from build123d import *

# Parameters (mm, degrees)
F1_DEPTH = 25
F3_R     = 2.1
F4_DEPTH = 25
F6_R     = 2.2
F7_DEPTH = 25
F8_R     = 4.99999


# Not quite as in the source:
# - a fillet or chamfer is up to 0.001 mm smaller than in the source, because OpenCascade refuses the exact size


with BuildPart() as f1:
    # F0 (on Right) → F1 (new body)
    with BuildSketch(Plane.YZ):
        Polygon((-127.7586124506, 10), (-127.7586124506, 0), (-18.2758603601, 0), (-18.2758603601, 50), (-28.2758603601, 50), (-28.2758603601, 10), align=None)
    extrude(amount=F1_DEPTH)

    # F3 (on face) → F4 (cut)
    with BuildSketch(Plane.XY.offset(10)):
        with Locations((12.5, -117.7586124506)):
            Circle(F3_R)
        with Locations((12.5, -42.7586124506)):
            Circle(F3_R)
    extrude(amount=-F4_DEPTH, mode=Mode.SUBTRACT)

    # F6 (on face) → F7 (cut)
    with BuildSketch(Plane.YZ.offset(25)):
        with Locations((-23.2758603601, 43)):
            Circle(F6_R)
        with Locations((-23.2758603601, 8)):
            Circle(F6_R)
    extrude(amount=-F7_DEPTH, mode=Mode.SUBTRACT)

    # F8 (radius 5 in the source; OpenCascade refuses exactly that, so slightly less here)
    f8_edges = [f1.edges().sort_by_distance(p)[0] for p in [
        (12.5, -28.27586, 10),
        (12.5, -18.27586, 50),
        (12.5, -28.27586, 50),
        (25, -127.758612, 5),
        (0, -127.758612, 5),
    ]]
    fillet(f8_edges, radius=F8_R)


solid = f1.part
Read the model definition and answer for the solid it produces. Units are mm, in the model's axes. A direction names the side the tool comes from. Coordinates: 2 decimals unless noted, no trailing zeros. Order: outer loops, then holes, each group sorted by start corner. A loop starts at its lowest first (then second) coordinate and runs counter-clockwise, first axis right, second up. Notation, with made-up numbers: M -12,56.25 L 24,56.25 A29 ccw 24,95.25 Z; hole C -3.5,57 d11. An arc over 180 degrees is marked long. Put each result on its own line as item: value. Start each with the question number.
Item 1: For faces 1 (the face through (12, -28.276, 30)), 2 (the face through (12, -127.759, 5)), determine the directions among +Z, -Z, +X, -X, +Y, -Y from which every point of the face is accessible in a straight line to the end or side of a thin tool.
Item 2: Section A-A, the plane x = 12.5 is taken. Count the separate pieces of the cut face and the enclosed holes in it, plus the area to 3 significant figures.
Item 3: Section B-B, the plane z = 7 is taken. Determine the outline of the cut face in (x, y), plus the area to 3 significant figures.
Item 4: Section C-C, the plane z = 43 is taken. Determine the outline of the cut face in (x, y).
Item 5: The mould has two halves that part along Y. Classify faces 3 (the face through (12, -74, 0)), 4 (the face through (10.95, -116.34, 5.07)), 5 (the face through (1.5, -126.33, 4.93)): +Y half, -Y half, draft (parallel to the pull), parting line (faces both ways), or undercut.
Item 6: Consider probe 1 along Z at (x, y) = (5.25, -23); probe 2 along Y at (x, z) = (12.5, 7.5); probe 3 along Z at (x, y) = (7.5, -25). Determine where each line is inside the solid, lowest interval first. Write a range as [from, to].
Item 7: Given pin 1 Ø5 at (x, z) = (7, 39) entering from -Y; pin 2 Ø1.5 at (y, z) = (-31, 13.5) entering from +X; pin 3 Ø6.5 at (x, y) = (12.5, -42.76) entering from +Z, each flat-ended and moving along its own axis, determine where each tip first touches the part or whether it passes through.
Computed:
1. face 1: +Z, +X, -X, -Y
1. face 2: +Z, -Z, +X, -X, -Y
2. separate pieces: 3
2. enclosed holes: 2
2. area: 1,380 mm2
3. outline: M 0,-122.76 A5 ccw 5,-127.76 L 20,-127.76 A5 ccw 25,-122.76 L 25,-25.24 L 0,-25.24 Z; M 0,-21.32 L 25,-21.32 L 25,-18.28 L 0,-18.28 Z; hole C 12.5,-117.76 d4.2; hole C 12.5,-42.76 d4.2
3. area: 2,600 mm2
4. outline: M 0,-28.28 L 25,-28.28 L 25,-25.48 L 0,-25.48 Z; M 0,-21.08 L 25,-21.08 L 25,-18.28 L 0,-18.28 Z
5. face 3: draft
5. face 4: undercut
5. face 5: -Y half
6. probe 1: z = [0, 5.82], [10.18, 40.82], [45.18, 49.99]
6. probe 2: y = [-127.76, -119.86], [-115.66, -44.86], [-40.66, -25.42], [-21.13, -18.28]
6. probe 3: z = [0, 6.63], [9.37, 41.63], [44.37, 49.69]
7. pin 1: stops at y = -28.28
7. pin 2: passes through
7. pin 3: stops at z = 10
